Part model, mm, in its own coordinate system. Give positions to 0.01 mm unless a question says otherwise; leave off trailing zeros. Write each loop counter-clockwise with the first axis right and the second up, starting at its lowest first coordinate (ties: lowest second). Pieces come first, ordered by that corner, then holes.
Autodesk Inventor part; units mm, degrees
ref_plane "Work Plane2" through (-12.5724, -12.5724, 0) normal (0.7071068, 0.7071068, 0) x (0, 0, 1)
ref_plane "XZ Plane" through (0, 0, 0) normal (0, 1, 0) x (-1, 0, 0)
ref_plane "XY Plane" through (0, 0, 0) normal (0, 0, 1) x (1, 0, 0)
ref_plane "Work Plane1" through (0, 0, 0) normal (0.7071068, 0.7071068, 0) x (0, 0, 1)
sketch "Sketch1" plane through (0, 0, 0) normal (1, 0, 0) x (0, 1, 0)
  circle A0 centre (0, 0) radius 19.05
  dimension "outerDiameter" = 38.1
ref_plane "Work Plane2" through (-12.5724, -12.5724, 0) normal (0.7071068, 0.7071068, 0) x (0, 0, 1)
extrude "Extrusion2" add sketch "Sketch1" against normal up to surface surface through (-12.5724, -12.5724, 0) normal (0.7071068, 0.7071068, 0)
sketch "Sketch3" plane through (0, 0, 0) normal (1, 0, 0) x (0, 0, -1)
  circle A0 centre (0, 0) radius 12.7
  dimension "thruHoleDiameter" = 25.4
extrude "Extrusion4" add sketch "Sketch3" against normal blind 93.853
sketch "Sketch4" plane through (-93.853, 0, 0) normal (-1, 0, 0) x (0, 0, 1)
  circle A0 centre (0, 0) radius 7.9375
  dimension "holeForString" = 15.875
extrude "Extrusion5" cut sketch "Sketch4" against normal through all
fillet "Fillet1" radius 2.54 3 edges at (0, 0, -7.9375) (-93.853, 0, -7.9375) (-93.853, 0, 12.7)
properties part number "ElectricFenceWasher"
1) Saw through at A-A (z = 0). Write the cut outline in (x, y).
Check result:
outline: (-93.85, -10.48) arc R2.54 ccw to (-91.33, -12.7) - (-12.44, -12.7) - (-6.09, -19.05) - (0, -19.05) - (0, -10.48) arc R2.54 ccw to (-2.54, -7.94) - (-91.31, -7.94) arc R2.54 ccw to start; (-93.85, 10.48) arc R2.54 ccw to (-91.31, 7.94) - (-2.54, 7.94) arc R2.54 ccw to (0, 10.48) - (0, 19.05) - (-44.19, 19.05) - (-37.84, 12.7) - (-91.33, 12.7) arc R2.54 ccw to start
2) Saw through at B-B (y = 0). Write the cut outline in (x, z).
Check result:
outline: (-93.85, -10.48) arc R2.54 ccw to (-91.33, -12.7) - (-25.14, -12.7) - (-25.14, -19.05) - (0, -19.05) - (0, -10.48) arc R2.54 ccw to (-2.54, -7.94) - (-91.31, -7.94) arc R2.54 ccw to start; (-93.85, 10.48) arc R2.54 ccw to (-91.31, 7.94) - (-2.54, 7.94) arc R2.54 ccw to (0, 10.48) - (0, 19.05) - (-25.14, 19.05) - (-25.14, 12.7) - (-91.33, 12.7) arc R2.54 ccw to start
3) Flat gauge pins, fed straight in: P1, Ø3, axis at x = -50, z = 9, coming from the -Y side; P2, Ø6, axis at x = -67.5, y = 9.5, coming from the +Z side; P3, Ø1, axis at x = -60, z = -8, coming from the +Y side. Where does each tip first touch, or does it go through?
Check result:
P1: stops at y = -10.25
P2: stops at z = 10.91
P3: stops at y = 10.25
4) Drill centre lines: L1, parallel to Y at x = -52, z = 0; L2, parallel to Y at x = -43, z = -1.5; L3, parallel to Y at x = -29.5, z = -1.5. Where is each one in solid material? Low to high.
Check result:
L1: y = -12.7 to -7.94, 7.94 to 12.7
L2: y = -12.61 to -7.79, 7.79 to 12.61, 17.86 to 18.99
L3: y = -12.61 to -7.79, 7.79 to 18.99
5) Mould opens along Z. For faces 1 (the cylindrical face through (-16.88, 18.17, 5.72)), 2 (the flat face through (0, -8, -8)), 3 (the cylindrical face through (-47.55, -7.75, -1.72)) say: +Z half, -Z half, draft (parallel to the pull), parting line (faces both ways), or undercut.
Check result:
face 1: parting line
face 2: draft
face 3: undercut
6) Saw through at D-D (z = 15.5). Write the cut outline in (x, y), and give its area (3 significant figures).
Check result:
outline: (-36.22, 11.07) - (-14.07, -11.07) - (0, -11.07) - (0, 11.07) - close
area: 557 mm2
7) Saw through at C-C (x = -57.5). Write the cut outline in (y, z) (1 decimal), and give its area (3 significant figures).
Check result:
outline: circle Ø25.4 at (0, 0); hole circle Ø15.9 at (0, 0)
area: 309 mm2
